Design review of the part built by this model. Coordinates are the model's own, in mm. Face numbers are marked on the shaded views. A direction names the side the tool comes from. Round coordinates to 2 decimals unless told otherwise and drop trailing zeros. Loops run counter-clockwise (first coordinate to the right, second up) from the corner with the lowest first, then second, coordinate; pieces in that order, holes last. Notation, with made-up numbers: (45.25, -33) - (104.25, -33) arc R10 cw to (104.25, -26) - close; hole circle Ø1 at (40.25, 8.25). An arc over 180 degrees is marked (long way). Answer as CSV lines item,"result". Start each with the question number.
(1) Consider section A-A (z = 0). Give the boundary of the cut face in (x, y).
(2) Consider section B-B (x = -160.5). Give the boundary of the cut face in (y, z), and give its area (3 significant figures).
(3) For the marked faces 1 and 2, list the 3-axis set-ups (+Z, -Z, +X, -X, +Y, -Y) from which the entire face can be reached by the end or side of a thin tool; tool diameter is ignored.
(4) Mouldability with a two-part tool opening along Y and no side actions: class the marked faces 3, 4 and 5 as released by +Y, released by -Y, zero draft, split by the parting line, or undercut.
(5) Consider section D-D (x = -108). Give the boundary of the cut face in (y, z), and give its area (3 significant figures).
(6) For P1, Ø12, axis at y = 35.5, z = -12.5, coming from the +X side; P2, Ø6, axis at y = 47.5, z = 15.5, coming from the -X side; P3, Ø1, axis at y = 3, z = 135, coming from the -X side, all flat-tipped, find the tip position at first contact; note any pin that passes through.
(7) Consider section C-C (y = 15). Give the boundary of the cut face in (x, z).
(8) Wall thickness on L1, parallel to Z at x = -100, y = 1; L2, parallel to Z at x = -18.5, y = 22; L3, parallel to X at y = 1.35, z = 0: over which ranges is each line inside the solid? List them lowest first.
Autodesk Inventor part; units mm, degrees
ref_plane "YZ Plane" through (0, 0, 0) normal (1, 0, 0) x (0, 1, 0)
ref_plane "XZ Plane" through (0, 0, 0) normal (0, 1, 0) x (-1, 0, 0)
ref_plane "XY Plane" through (0, 0, 0) normal (0, 0, 1) x (1, 0, 0)
sketch "Szkic1" plane through (0, 0, 0) normal (0, 0, 1) x (1, 0, 0)
  line L0 (0, 0) -> (-200, 0)
  line L1 (0, 0) -> (0, 120)
  line L2 (0, 120) -> (-200, 0)
  dimension "d0" = 200
  dimension "d1" = 120
extrude "Wyciągnięcie proste1" add sketch "Szkic1" along normal mid plane 300
shell "Skorupa1" thickness 4 removed faces 1 at (0, 40, -50)
sketch "Szkic2" plane through (-185.5587, 4, -146) normal (0, 1, 0) x (1, 0, 0)
  line L0 (68.5587, -133.5) -> (102.5587, -133.5)
  line L1 (102.5587, -133.5) -> (102.5587, -158.5)
  line L2 (102.5587, -158.5) -> (68.5587, -158.5)
  line L3 (68.5587, -158.5) -> (68.5587, -133.5)
  line L4 (185.5587, 4) -> (-14.4413, 4)
  line L5 (185.5587, 4) -> (185.5587, -296)
  circle A0 centre (85.5587, -146) radius 11.5
  point P0 (185.5587, -146)
  dimension "d5" = 34
  dimension "d6" = 25
  dimension "d7" = 137.5
  dimension "d8" = 83
  dimension "d9" = 23
  dimension "d10" = 100
  dimension "d11" = 150
extrude "Wyciągnięcie proste2" cut sketch "Szkic2" against normal through all contours A0
extrude "Wyciągnięcie proste3" cut sketch "Szkic2" against normal blind 2
sketch "Szkic3" plane through (-200, 0, 150) normal (0, -1, 0) x (1, 0, 0)
  circle A0 centre (100, -150) radius 11.5
  line L0 (200, -300) -> (200, 0)
  line L1 (0, 0) -> (200, 0)
  line L2 (0, 0) -> (0, -300)
  line L3 (200, -300) -> (0, -300)
  line L4 (155.5, -159.75) -> (170, -159.75)
  line L5 (170, -159.75) -> (170, -140.25)
  line L6 (170, -140.25) -> (155.5, -140.25)
  line L7 (155.5, -140.25) -> (155.5, -159.75)
  line L8 (155.5, -159.75) -> (170, -140.25) construction
  line L9 (170, -159.75) -> (155.5, -140.25) construction
  line L10 (170, -143.25) -> (155.5, -143.25)
  point P0 (200, -150)
  point P1 (162.75, -150)
  dimension "d16" = 14.5
  dimension "d17" = 19.5
  dimension "d18" = 140.25
  dimension "d19" = 30
  dimension "d20" = 3
extrude "Wyciągnięcie proste4" cut sketch "Szkic3" against normal blind 2 contours L7 L10 L5 L4
extrude "Wyciągnięcie proste5" cut sketch "Szkic3" against normal blind 4 contours L7 L6 L5 L10
sketch "Szkic4" plane through (-185.5587, 4, -146) normal (0, 1, 0) x (1, 0, 0)
  line L0 (141.0587, -152.75) -> (155.5587, -152.75)
  line L1 (155.5587, -152.75) -> (155.5587, -155.75)
  line L2 (155.5587, -155.75) -> (141.0587, -155.75)
  line L3 (141.0587, -155.75) -> (141.0587, -152.75)
  line L4 (102.5587, -133.5) -> (102.5587, -158.5)
  line L5 (102.5587, -158.5) -> (68.5587, -158.5)
  line L6 (68.5587, -158.5) -> (68.5587, -133.5)
  line L7 (68.5587, -133.5) -> (102.5587, -133.5)
  line L8 (185.5587, 0) -> (185.5587, -292)
  line L9 (185.5587, 0) -> (0, 0)
  line L10 (0, -292) -> (0, 0)
  line L11 (0, -292) -> (185.5587, -292)
  line L12 (81.5587, -158.5) -> (89.5587, -158.5)
  line L13 (89.5587, -158.5) -> (89.5587, -222)
  line L14 (89.5587, -292) -> (81.5587, -292)
  line L15 (81.5587, -222) -> (81.5587, -158.5)
  line L16 (141.0587, -155.75) -> (155.5587, -155.75)
  line L17 (155.5587, -292) -> (141.0587, -292)
  line L18 (142.3087, -155.75) -> (154.3087, -155.75)
  line L19 (154.3087, -155.75) -> (154.3087, -222)
  line L20 (154.3087, -292) -> (142.3087, -292)
  line L21 (142.3087, -222) -> (142.3087, -155.75)
  line L22 (109.3319, -242) -> (124.3319, -242)
  line L23 (124.3319, -242) -> (124.3319, -292)
  line L24 (124.3319, -292) -> (109.3319, -292)
  line L25 (109.3319, -292) -> (109.3319, -242)
  line L26 (109.3319, -242) -> (109.5587, -242)
  line L27 (124.3319, -242) -> (122.3087, -242)
  line L28 (109.3319, -257) -> (116.5587, -257)
  line L29 (124.3319, -257) -> (119.3087, -257)
  arc A0 (89.5587, -222) -> (109.5587, -242) centre (109.5587, -222) ccw
  arc A1 (81.5587, -222) -> (116.5587, -257) centre (116.5587, -222) ccw
  arc A2 (122.3087, -242) -> (142.3087, -222) centre (122.3087, -222) ccw
  arc A3 (119.3087, -257) -> (154.3087, -222) centre (119.3087, -222) ccw
  line L30 (124.3319, -257) -> (124.3319, -256.6377)
  point P0 (185.5587, -146)
  point P1 (124.3319, -267)
  point P2 (116.8319, -292)
  point P3 (142.3087, -242)
  point P4 (89.5587, -257)
  point P5 (142.3087, -257)
  point P6 (109.3319, -256.2458)
  dimension "d25" = 96
  dimension "d26" = 8
  dimension "d28" = 31.25
  dimension "d29" = 12
  dimension "d33" = 15
  dimension "d34" = 61.2269
  dimension "d36" = 50
  dimension "d37" = 30
  dimension "d38" = 30
  dimension "d39" = 44.5
  dimension "d40" = 35
  dimension "d41" = 20
  dimension "d42" = 35
  dimension "d43" = 20
  dimension "d44" = 35
extrude "Wyciągnięcie proste6" cut sketch "Szkic4" against normal blind 2 contours L2 L19 A3 L23 L22 A2 L21 | L22 L23 A3 L29 L11 L25 L28 A1 | L23 L29 A3 | L25 A1 L15 L5 L13 A0 | A1 L28 L25
properties part number "PitchedRoof"
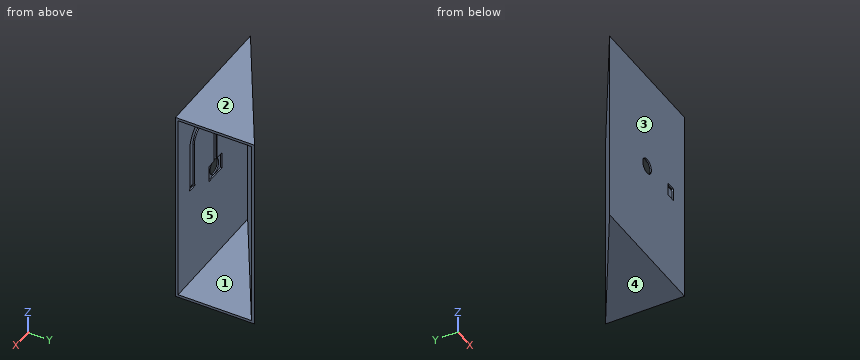
Determined:
1,outline,"(-200, 0) - (-111.5, 0) - (-111.5, 2) - (-117, 2) - (-117, 4) - (-185.56, 4) - (0, 115.34) - (0, 120) - close; (-88.5, 0) - (-44.5, 0) - (-44.5, 2) - (-30, 2) - (-30, 0) - (0, 0) - (0, 4) - (-83, 4) - (-83, 2) - (-88.5, 2) - close"
2,outline,"(0, -150) - (23.7, -150) - (23.7, 150) - (0, 150) - close; hole (4, -146) - (19.04, -146) - (19.04, 146) - (4, 146) - close"
2,area,"2,720 mm^2"
3,face 1,"+X"
3,face 2,"+Z, +X, -X, +Y, -Y"
4,face 3,"released by -Y"
4,face 4,"zero draft"
4,face 5,"undercut"
5,outline,"(0, -150) - (55.2, -150) - (55.2, 150) - (0, 150) - (0, 8.26) - (2, 8.26) - (2, 12.5) - (4, 12.5) - (4, 146) - (50.54, 146) - (50.54, -146) - (4, -146) - (4, -12.5) - (2, -12.5) - (2, -8.26) - (0, -8.26) - close"
5,area,"2,890 mm^2"
6,P1,"stops at x = -123.06"
6,P2,"stops at x = -125.83"
6,P3,"stops at x = -195.83"
7,outline,"(-175, -150) - (0, -150) - (0, -146) - (-167.23, -146) - (-167.23, 146) - (0, 146) - (0, 150) - (-175, 150) - close"
8,L1,"z = -150 to -11.5, 11.5 to 150"
8,L2,"z = -150 to -146, 146 to 150"
8,L3,"x = -197.75 to -111.5, -88.5 to -44.5, -30 to 0"
